```python
from build123d import *

# Parameters (mm, degrees)
F1_DEPTH = 203.2
F3_D     = 4.7625
F5_D     = 4.7625


with BuildPart() as f1:
    # F0 (on Front) → F1 (new body)
    with BuildSketch(Plane.XZ):
        with BuildLine():
            Line((0, -38.1), (0, 0))
            Line((0, 0), (-38.1, 0))
            Line((-38.1, 0), (-38.1, -1.5875))
            ThreePointArc((-38.1, -1.5875), (-37.635032, -2.710032), (-36.5125, -3.175))
            Line((-36.5125, -3.175), (-4.7625, -3.175))
            ThreePointArc((-4.7625, -3.175), (-3.639968, -3.639968), (-3.175, -4.7625))
            Line((-3.175, -4.7625), (-3.175, -36.5125))
            ThreePointArc((-3.175, -36.5125), (-2.710032, -37.635032), (-1.5875, -38.1))
            Line((-1.5875, -38.1), (0, -38.1))
        make_face()
    extrude(amount=F1_DEPTH)

    # F3 (through all)
    with Locations(Plane.XY):
        with Locations((-19.05, -177.8), (-28.575, -101.6), (-19.05, -25.4)):
            Hole(F3_D / 2)

    # F5 (through all)
    with Locations(Plane.YZ):
        with Locations((-25.4, -19.05), (-101.6, -28.575), (-177.8, -19.05)):
            Hole(F5_D / 2)


solid = f1.part
```
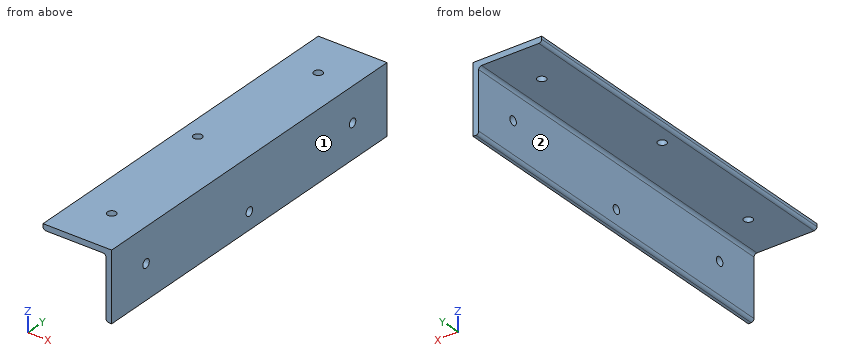
Design review of the part built by this model. Coordinates are the model's own, in mm. Face numbers are marked on the shaded views. A direction names the side the tool comes from. Coordinates: 2 decimals unless noted, no trailing zeros. Loops run counter-clockwise (first coordinate to the right, second up) from the corner with the lowest first, then second, coordinate; pieces in that order, holes last. Notation, with made-up numbers: (73.25, 4) -> (94.25, 4) arc R25 ccw to (94.25, 17) -> close; hole circle Ø5 at (77.25, 20.25). An arc over 180 degrees is marked (long way). Answer as a JSON object with one key per item and string values.
Q1. Take a section at A-A on x = -19.05. Give the boundary of the cut face in (y, z) (3 decimals).
Answer block:
{"outline": "(-203.2, -3.175) -> (-180.181, -3.175) -> (-180.181, 0) -> (-203.2, 0) -> close; (-175.419, -3.175) -> (-27.781, -3.175) -> (-27.781, 0) -> (-175.419, 0) -> close; (-23.019, -3.175) -> (0, -3.175) -> (0, 0) -> (-23.019, 0) -> close"}
Q2. Take a section at D-D on z = -34. Give the boundary of the cut face in (x, y) (3 decimals).
Answer block:
{"outline": "(-3.175, -203.2) -> (0, -203.2) -> (0, 0) -> (-3.175, 0) -> close"}
Q3. Clearance check with flat-ended pins moving along their axes: pin 1 Ø8 at (x, y) = (-11.5, -178.5) entering from -Z (3 decimals); pin 2 Ø12 at (y, z) = (-133.5, -26) entering from -X (3 decimals). State where each tip first meets the part, or that it passes through.
Answer block:
{"pin 1": "stops at z = -3.175", "pin 2": "stops at x = -3.175"}
Q4. Tool access review of the marked faces 1 and 2: name each direction out of +Z, -Z, +X, -X, +Y, -Y from which nothing blocks a thin tool from reaching the whole face with its end or side.
Answer block:
{"face 1": "+Z, -Z, +X, +Y, -Y", "face 2": "-Z, -X, +Y, -Y"}
Q5. To check wall thickness, follow L1, parallel to X at y = -177.8, z = -1.3; L2, parallel to Y at x = -19, z = -1; L3, parallel to Z at x = -0.7, y = -101.6. State the ranges of each line that lie inside material, in increasing order.
Answer block:
{"L1": "x = -38.1 to -21.43, -16.67 to 0", "L2": "y = -203.2 to -180.18, -175.42 to -27.78, -23.02 to 0", "L3": "z = -38.1 to -30.96, -26.19 to 0"}
Q6. Take a section at C-C on y = -159. Give the boundary of the cut face in (x, z) (1 decimal), plus the area to 3 significant figures.
Answer block:
{"outline": "(-38.1, -1.6) arc R1.6 ccw to (-36.5, -3.2) -> (-4.8, -3.2) arc R1.6 cw to (-3.2, -4.8) -> (-3.2, -36.5) arc R1.6 ccw to (-1.6, -38.1) -> (0, -38.1) -> (0, 0) -> (-38.1, 0) -> close", "area": "231 mm^2"}
Q7. Take a section at B-B on y = -25.4. Give the boundary of the cut face in (x, z) (1 decimal).
Answer block:
{"outline": "(-38.1, -1.6) arc R1.6 ccw to (-36.5, -3.2) -> (-21.4, -3.2) -> (-21.4, 0) -> (-38.1, 0) -> close; (-16.7, -3.2) -> (-4.8, -3.2) arc R1.6 cw to (-3.2, -4.8) -> (-3.2, -16.7) -> (0, -16.7) -> (0, 0) -> (-16.7, 0) -> close; (-3.2, -36.5) arc R1.6 ccw to (-1.6, -38.1) -> (0, -38.1) -> (0, -21.4) -> (-3.2, -21.4) -> close"}
